Geometry check sheet. Reference: the model listing, model coordinates, mm. A direction names the side the tool comes from. Coordinates: 2 decimals unless noted, no trailing zeros. Write each loop counter-clockwise with the first axis right and the second up, starting at its lowest first coordinate (ties: lowest second). Pieces come first, ordered by that corner, then holes. Notation, with made-up numbers: M 59.5,69 L 103.5,69 A23 ccw 103.5,107 Z; hole C 43,-8.75 d6. An arc over 180 degrees is marked long. Answer as a JSON object with one key per item and string values. Group by question number.
```python
from build123d import *

# Parameters (mm, degrees)
SKETCH2_R           = 10
SKETCH2_R_2         = 6.75
BOSS_EXTRUDE1_DEPTH = 34
SKETCH3_W           = 20
SKETCH3_H           = 20
BOSS_EXTRUDE2_DEPTH = 24
CUT_EXTRUDE1_DEPTH  = 24
SKETCH5_R           = 4
CUT_EXTRUDE2_DEPTH  = 63.161081072


with BuildPart() as part:
    # Sketch2 → Boss-Extrude1 (new body)
    with BuildSketch(Plane(origin=(0, 0, 0), x_dir=(1, 0, 0), z_dir=(0, 1, 0))):
        with Locations(Location((0, 0, 0), (0, 0, 270))):
            Circle(SKETCH2_R)
        with Locations(Location((0, 0, 0), (0, 0, 270))):
            Circle(SKETCH2_R_2, mode=Mode.SUBTRACT)
    extrude(amount=-BOSS_EXTRUDE1_DEPTH)

    # Sketch3 → Boss-Extrude2 (add)
    with BuildSketch(Plane.XZ.offset(34)):
        Rectangle(SKETCH3_W, SKETCH3_H)
    extrude(amount=BOSS_EXTRUDE2_DEPTH)

    # Sketch4 → Cut-Extrude1 (cut, symmetric)
    with BuildSketch(Plane.XY):
        with BuildLine():
            Line((-10, -58), (0, -58))
            ThreePointArc((0, -58), (-7.071067812, -55.071067812), (-10, -48))
            Line((-10, -48), (-10, -58))
        make_face()
    cut_extrude1 = extrude(amount=CUT_EXTRUDE1_DEPTH, both=True, mode=Mode.SUBTRACT)

    # Mirror1: Cut-Extrude1 across plane
    add(cut_extrude1.mirror(Plane(origin=(0, 0, 0), x_dir=(0, 0, 1), z_dir=(1, 0, 0))), mode=Mode.SUBTRACT)

    # Sketch5 → Cut-Extrude2 (cut, through all)
    with BuildSketch(Plane(origin=(0, 0, -10), x_dir=(-1, 0, 0), z_dir=(0, 0, -1))):
        with Locations((0, -48)):
            Circle(SKETCH5_R)
    extrude(amount=-CUT_EXTRUDE2_DEPTH, mode=Mode.SUBTRACT)


solid = part.part
```
1) Section check A-A (z = -1.25). Record the cut outline in (x, y).
2) Go/stop test with flat-tipped pins: pin 1 Ø4 at (x, z) = (2.5, 2) entering from +Y; pin 2 Ø2 at (x, y) = (-4.5, -12) entering from +Z; pin 3 Ø8 at (y, z) = (-10, 6.5) entering from -X. Record where each tip stops, or that it passes through.
3) Section check D-D (x = 5). Record the cut outline in (y, z), then the cut area to 3 significant figures.
4) Set-up check for faces 1 (the flat face through (8, -34, 8)), 2 (the flat face through (-8, -34, 8)), 3 (the flat face through (0, -34, 0)), 4 (the flat face through (-8, -34, -8)), 5 (the flat face through (0, -43, -10)): record each of +Z, -Z, +X, -X, +Y, -Y from which the full face is reachable in a straight line by a thin tool's end or side.
5) Section check C-C (y = -21). Record the cut outline in (x, z).
6) Material ranges on probe 1 along X at (y, z) = (-9, 0); probe 2 along Y at (x, z) = (0.25, -8.25); probe 3 along Y at (x, z) = (0, -3.75), recorded low to high. Write a range as [from, to].
7) Draft check along X on faces 6 (the cylindrical face through (-9.76, -16.76, -2.17)), 7 (the flat face through (8, -34, -8)), 8 (the cylindrical face through (-6.59, -16.76, -1.46)). Enter one of: +X half, -X half, draft (parallel to the pull), parting line (faces both ways), or undercut.
8) Section check B-B (y = -51). Record the cut outline in (x, z), then the cut area to 3 significant figures.
Entries:
{
 "1": {"outline": "M -10,-48 A10 ccw 10,-48 L 10,-34 L 9.92,-34 L 9.92,0 L 6.63,0 L 6.63,-34 L -6.63,-34 L -6.63,0 L -9.92,0 L -9.92,-34 L -10,-34 Z; hole C 0,-48 d8"},
 "2": {"pin 1": "y = -34", "pin 2": "z = 9.37", "pin 3": "x = -9.68"},
 "3": {"outline": "M -56.66,-10 L -34,-10 L -34,-8.66 L 0,-8.66 L 0,-4.53 L -34,-4.53 L -34,4.53 L 0,4.53 L 0,8.66 L -34,8.66 L -34,10 L -56.66,10 Z", "area": "734 mm^2"},
 "4": {"face 1": "+Z, +X, +Y", "face 2": "+Z, -X, +Y", "face 3": "+Y", "face 4": "-Z, -X, +Y", "face 5": "-Z, +X, -X, +Y, -Y"},
 "5": {"outline": "C 0,0 d20; hole C 0,0 d13.5"},
 "6": {"probe 1": "[-10, -6.75], [6.75, 10]", "probe 2": "[-58, -51.99], [-44.01, 0]", "probe 3": "[-58, -52], [-44, -34]"},
 "7": {"face 6": "parting line", "face 7": "draft", "face 8": "undercut"},
 "8": {"outline": "M -9.54,-10 L -2.65,-10 L -2.65,10 L -9.54,10 Z; M 2.65,-10 L 9.54,-10 L 9.54,10 L 2.65,10 Z", "area": "276 mm^2"}
}
